The listing builds one solid part. Answer for the finished solid, in the listing's coordinates (mm). Coordinates: 2 decimals unless noted, no trailing zeros. Order: outer loops, then holes, each group sorted by start corner. A loop starts at its lowest first (then second) coordinate and runs counter-clockwise, first axis right, second up.
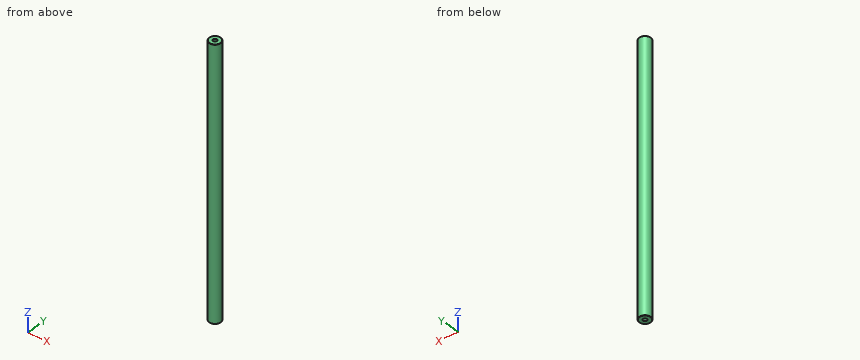
```python
from build123d import *

# Parameters (mm, degrees)
SKETCH_1_R      = 5
EXTRUDE_1_DEPTH = 115
CHAMFER_1_SIZE  = 0.2


with BuildPart() as part:
    # ｽｹｯﾁ1 → ﾎﾞｽ - 押し出し1 (new, symmetric)
    with BuildSketch(Plane.XY):
        Circle(SKETCH_1_R)
    extrude(amount=EXTRUDE_1_DEPTH, both=True)

    # ｽｹｯﾁ3 → M4x0.7 ねじ穴1 (revolve, cut)
    with BuildSketch(Plane(origin=(0, 0, 115), x_dir=(0, -1, 0), z_dir=(1, 0, 0))):
        Polygon((0, 0), (0, 12.491420021), (1.65, 11.5), (1.65, 0), align=None)
    m4x0_7_1 = revolve(axis=Axis((0, 0, 121.35), (0, 0, -1)), mode=Mode.SUBTRACT)

    # ﾐﾗｰ1: M4x0.7 ねじ穴1 across plane
    add(m4x0_7_1.mirror(Plane.XY), mode=Mode.SUBTRACT)

    # 面取り1
    chamfer_1_edges = [part.edges().sort_by_distance(p)[0] for p in [
        (-5, 0, -115),
        (-5, 0, 115),
    ]]
    chamfer(chamfer_1_edges, length=CHAMFER_1_SIZE)


solid = part.part
```
(1) Each of these flat-tipped pins is pushed along its axis until it touches: pin 1 Ø6 at (x, z) = (-3.5, 85.5) entering from -Y; pin 2 Ø3 at (x, y) = (0, 0) entering from +Z; pin 3 Ø1 at (x, z) = (2.5, -58.5) entering from +Y. Where does it stop, or does it pass through?
(2) Find section A-A (z = 82). Write down the section's boundary in (x, y).
(3) Consider line 1 (Y direction, x = 0, z = -109); line 2 (X direction, y = 0.25, z = 15); line 3 (Z direction, x = -1, y = -1.25). Determine where each line is inside the solid, lowest interval first.
Findings below:
1. pin 1: stops at y = -4.97
1. pin 2: stops at z = 103.41
1. pin 3: stops at y = 4.58
2. outline: circle Ø10 at (0, 0)
3. line 1: y = -5 to -1.65, 1.65 to 5
3. line 2: x = -4.99 to 4.99
3. line 3: z = -103.47 to 103.47
